Source: CAD feature listing. Evaluate the final solid. Frame: model axes, mm. Coordinates: 2 decimals unless noted, no trailing zeros. Write each loop counter-clockwise with the first axis right and the second up, starting at its lowest first coordinate (ties: lowest second). Pieces come first, ordered by that corner, then holes. Notation, with made-up numbers: (57, 81) - (93, 81) arc R10 cw to (93, 98) - close; hole circle Ø10 at (46.25, 25.25). An arc over 180 degrees is marked (long way). One line per question, with ' | ' between items. Start each with the question number.
Q1. Contact query for a flat-ended pin moving along its axis: P1, Ø5, axis at x = -13.5, z = -1, coming from the +Y side. Output: stop coordinate, or through.
Q2. Draft query along X for faces 1 (the face through (30, 9, 0)), 2 (the face through (-27.578, 4.662, 0.49)), 3 (the face through (0, 9, 35)). Return one class per face: +X half, -X half, draft (parallel to the pull), parting line (faces both ways), or undercut.
Q3. Line query: line 1 (X direction, y = 5, z = 2.5); line 2 (Y direction, x = -25, z = -28); line 3 (Z direction, x = -12.5, y = 12.5). Output: solid intervals per line, ascending.
Q4. Cut plane B-B, the plane x = -24. Return loops of the section in (y, z), plus the area to 3 significant figures.
Q5. Cut plane A-A, the plane y = 5. Return loops of the section in (x, z), plus the area to 3 significant figures.
Q6. Cut plane C-C, the plane z = -19.5. Return loops of the section in (x, y), plus the area to 3 significant figures.
Q7. Cut plane D-D, the plane y = 14.5. Return loops of the section in (x, z), plus the area to 3 significant figures.
Autodesk Inventor part; units mm, degrees
ref_plane "YZ Plane" through (0, 0, 0) normal (1, 0, 0) x (0, 1, 0)
ref_plane "XZ Plane" through (0, 0, 0) normal (0, 1, 0) x (-1, 0, 0)
ref_plane "XY Plane" through (0, 0, 0) normal (0, 0, 1) x (1, 0, 0)
sketch "Sketch1" plane through (0, 0, 0) normal (0, 1, 0) x (-1, 0, 0)
  line L0 (-30, 35) -> (30, 35)
  line L1 (30, 35) -> (30, -35)
  line L2 (30, -35) -> (-30, -35)
  line L3 (-30, -35) -> (-30, 35)
  line L4 (-30, 35) -> (30, -35) construction
  line L5 (30, 35) -> (-30, -35) construction
  point P0 (0, 0)
  dimension "d0" = 60
  dimension "d1" = 70
extrude "Extrusion1" add sketch "Sketch1" along normal blind 18
sketch "Sketch2" plane through (30, 0, -35) normal (0, 0, -1) x (-1, 0, 0)
  line L0 (0, 0) -> (60, 0)
  line L1 (60, 0) -> (60, 18)
  line L2 (0, 18) -> (60, 18)
  line L3 (0, 0) -> (0, 18)
  line L4 (0, 5) -> (60, 5) construction
  line L5 (30, 0) -> (30, 18) construction
  line L6 (0, 18) -> (60, 18)
  point P0 (5, 5)
  point P1 (30, 5)
  point P2 (55, 5)
  dimension "d4" = 5
  dimension "d6" = 5
hole "Hole1" at (25, 5, -35) at (0, 5, -35) at (-25, 5, -35) direction (0, 0, 1) diameter 5.2 end through all
sketch "Sketch3" plane through (30, 0, 35) normal (1, 0, 0) x (0, 0, -1)
  line L0 (0, 2.4) -> (70, 2.4)
  line L1 (0, 2.4) -> (0, 7.6)
  line L2 (70, 7.6) -> (70, 2.4)
  line L3 (0, 7.6) -> (70, 7.6)
  line L4 (0, 0) -> (70, 0)
  line L5 (70, 0) -> (70, 18)
  line L6 (0, 18) -> (70, 18)
  line L7 (0, 0) -> (0, 18)
  circle A0 centre (35, 28) radius 18
  point P0 (35, 0)
  point P1 (35, 0)
  point P2 (49.9666, 18)
  point P3 (20.0334, 18)
  dimension "d14" = 36
  dimension "d15" = 10
extrude "Extrusion2" cut sketch "Sketch3" against normal through all contours L6 A0 picked at (30.9706, 16.8877)
sketch "Sketch4" plane through (0, 18, 0) normal (0, 1, 0) x (1, 0, 0)
  line L0 (-22.4, -35) -> (-27.6, -35)
  line L1 (-27.6, 35) -> (-22.4, 35)
  line L2 (2.6, -35) -> (-2.6, -35)
  line L3 (-2.6, 35) -> (2.6, 35)
  line L4 (27.6, -35) -> (22.4, -35)
  line L5 (22.4, 35) -> (27.6, 35)
  line L6 (-30, -35) -> (30, -35)
  line L7 (-12.5, -35) -> (-12.5, 35) construction
  line L8 (2.6, 35) -> (22.4, 35)
  line L9 (2.6, -35) -> (2.6, 35)
  line L10 (-22.4, 35) -> (-2.6, 35)
  line L11 (-22.4, -35) -> (-22.4, 35)
  line L12 (12.5, 35) -> (12.5, -35) construction
  line L13 (-30, -14.9666) -> (-30, -35)
  line L14 (-30, 35) -> (-30, 14.9666)
  line L15 (-30, 24.9833) -> (10, 24.9833) construction
  line L16 (-30, -24.9833) -> (30, -24.9833) construction
  line L17 (30, -35) -> (30, -14.9666)
  point P0 (0, 0)
  point P1 (-12.5, -24.9833)
  point P2 (12.5, -24.9833)
  point P3 (12.5, 24.9833)
  point P4 (-12.5, 24.9833)
hole "Hole2" at (-12.5, 18, 24.9833) at (12.5, 18, 24.9833) at (12.5, 18, -24.9833) at (-12.5, 18, -24.9833) direction (0, -1, 0) diameter 3.2 end through all
properties part number "18_Kep_han_A" material "ABS Plastic"
Reply:
1) P1: stops at y = 10.34
2) face 1: +X half | face 2: undercut | face 3: draft
3) line 1: x = -30 to -27.6, -22.4 to -2.6, 2.6 to 22.4, 27.6 to 30 | line 2: y = 0 to 2.4, 7.6 to 18 | line 3: z = -35 to -26.58, -23.38 to -9.15, 9.15 to 23.38, 26.58 to 35
4) outline: (0, -35) - (2.6, -35) - (2.6, 35) - (0, 35) - close; (7.4, -35) - (18, -35) - (18, -14.97) arc R18 cw to (18, 14.97) - (18, 35) - (7.4, 35) - close | area: 756 mm^2
5) outline: (-30, -35) - (-27.6, -35) - (-27.6, 35) - (-30, 35) - close; (-22.4, -35) - (-2.6, -35) - (-2.6, 35) - (-22.4, 35) - close; (2.6, -35) - (22.4, -35) - (22.4, 35) - (2.6, 35) - close; (27.6, -35) - (30, -35) - (30, 35) - (27.6, 35) - close; hole circle Ø3.2 at (-12.5, -24.98); hole circle Ø3.2 at (-12.5, 24.98); hole circle Ø3.2 at (12.5, -24.98); hole circle Ø3.2 at (12.5, 24.98) | area: 3,080 mm^2
6) outline: (-30, 0) - (30, 0) - (30, 18) - (-30, 18) - close; hole circle Ø5.2 at (-25, 5); hole circle Ø5.2 at (0, 5); hole circle Ø5.2 at (25, 5) | area: 1,020 mm^2
7) outline: (-30, -35) - (30, -35) - (30, -11.91) - (-30, -11.91) - close; (-30, 11.91) - (30, 11.91) - (30, 35) - (-30, 35) - close; hole circle Ø3.2 at (-12.5, -24.98); hole circle Ø3.2 at (-12.5, 24.98); hole circle Ø3.2 at (12.5, -24.98); hole circle Ø3.2 at (12.5, 24.98) | area: 2,740 mm^2
